from build123d import *

# Parameters (mm, degrees)
SKETCH3_R          = 250
CUT_EXTRUDE7_DEPTH = 2
SKETCH6_R          = 2
CUT_EXTRUDE8_DEPTH = 498
SKETCH7_R          = 100
CUT_EXTRUDE9_DEPTH = 2


with BuildPart() as part:
    # Sketch2 → Revolve2 (revolve)
    with BuildSketch(Plane.XY):
        Polygon((0, 0), (0, -252), (500, -102), (500, 0), align=None)
        Polygon((2, -249.311938698), (498, -100.511938698), (498, -2), (2, -2), align=None, mode=Mode.SUBTRACT)
    revolve(axis=Axis((0, 0, 0), (1, 0, 0)))

    # Sketch3 → Cut-Extrude7 (cut)
    with BuildSketch(Plane.ZY):
        Circle(SKETCH3_R)
    extrude(amount=-CUT_EXTRUDE7_DEPTH, mode=Mode.SUBTRACT)

    # Sketch6 → Cut-Extrude8 (cut)
    with BuildSketch(Plane.ZY.offset(-2)):
        Circle(SKETCH6_R)
    extrude(amount=-CUT_EXTRUDE8_DEPTH, mode=Mode.SUBTRACT)

    # Sketch7 → Cut-Extrude9 (cut)
    with BuildSketch(Plane(origin=(500, 0, 0), x_dir=(0, 0, -1), z_dir=(1, 0, 0))):
        Circle(SKETCH7_R)
    extrude(amount=-CUT_EXTRUDE9_DEPTH, mode=Mode.SUBTRACT)


solid = part.part
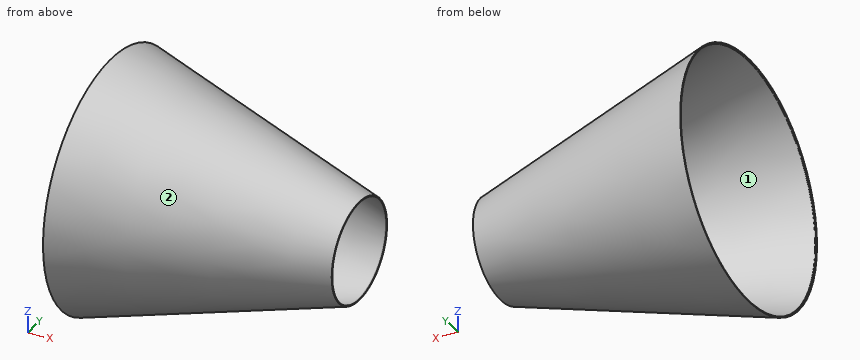
Geometry check sheet. Reference: the model listing, model coordinates, mm. Face numbers are marked on the shaded views. Coordinates: 2 decimals unless noted, no trailing zeros. Order: outer loops, then holes, each group sorted by start corner. A loop starts at its lowest first (then second) coordinate and runs counter-clockwise, first axis right, second up. Notation, with made-up numbers: (-35, 31.5) - (-29, 31.5) arc R14 cw to (-29, 56.5) - close; hole circle Ø1 at (59, -33.75). An arc over 180 degrees is marked (long way). Answer in a Markdown table with one row per item. Add a question column.
1) Release check for a two-part mould opening along Y. For the marked faces 1 and 2 record: +Y half, -Y half, draft (parallel to the pull), parting line (faces both ways), or undercut.
2) Material ranges on line 1 along Y through (x, z) = (498.5, 0); line 2 along Y through (x, z) = (199, -46); line 3 along Z through (x, y) = (233, -87), recorded low to high. Write a range as [from, to].
3) Cross-section at D-D, the plane x = 405. Record the cut outline in (y, z).
4) Cross-section at A-A, the plane z = 0. Record the cut outline in (x, y), then the cut area to 3 significant figures.
5) Gauge pin test, flat ends, axial feed: P1, Ø4, axis at x = 250, y = 123.5, coming from the -Z side; P2, Ø2, axis at x = 66, y = 50.5, coming from the +Z side; P3, Ø2, axis at x = 311.5, z = 55, coming from the +Y side. Record the tip position at first contact, or that the pin passes through.
6) Cross-section at C-C, the plane x = 145.5. Record the cut outline in (y, z).
Check result:
| question | item | result |
|---|---|---|
| 1 | face 1 | undercut |
| 1 | face 2 | parting line |
| 2 | line 1 | y = [-102.45, -100], [100, 102.45] |
| 2 | line 2 | y = [-186.72, -184.57], [184.57, 186.72] |
| 2 | line 3 | z = [-159.97, -157.59], [157.59, 159.97] |
| 3 | outline | circle Ø261 at (0, 0); hole circle Ø256.82 at (0, 0) |
| 4 | outline | (0, -252) - (500, -102) - (500, -100) - (498, -100) - (498, -100.51) - (2, -249.31) - (2, -250) - (0, -250) - close; (0, 250) - (2, 250) - (2, 249.31) - (498, 100.51) - (498, 100) - (500, 100) - (500, 102) - (0, 252) - close |
| 4 | area | 2,090 mm² |
| 5 | P1 | stops at z = -128.88 |
| 5 | P2 | stops at z = 227.02 |
| 5 | P3 | stops at y = 149.19 |
| 6 | outline | circle Ø416.7 at (0, 0); hole circle Ø412.52 at (0, 0) |
